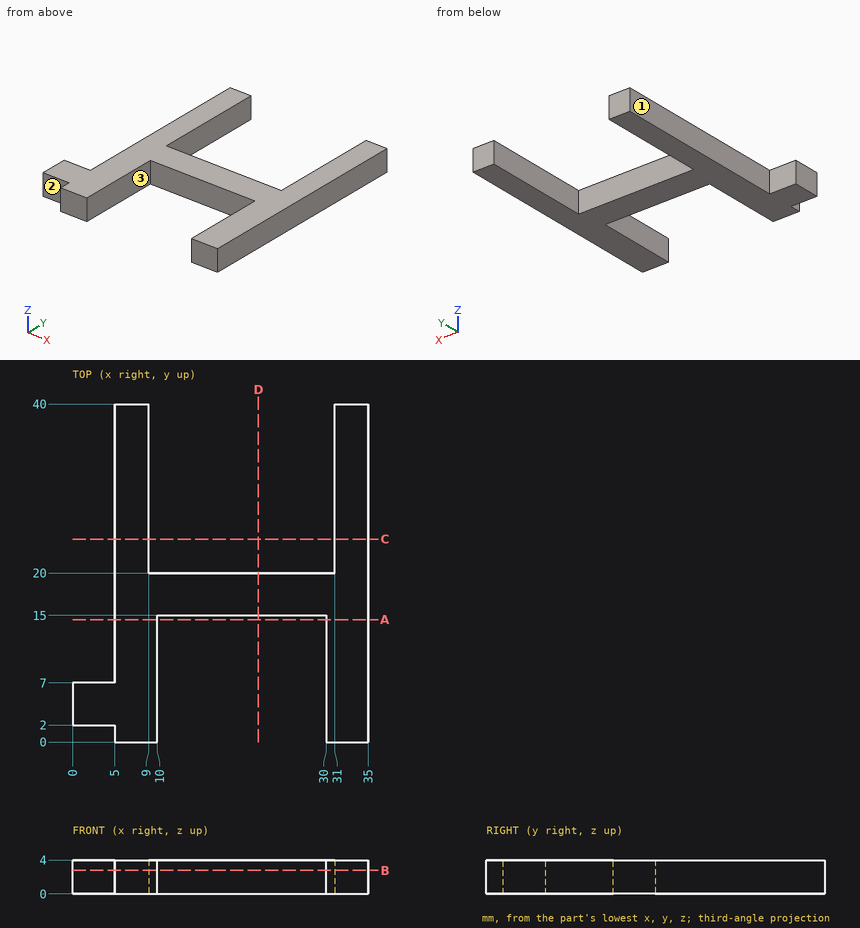
Drawing for the job (mm, zero at the part's lowest x, y, z). A direction names the side the tool comes from. Round coordinates to 2 decimals unless told otherwise and drop trailing zeros. Loops run counter-clockwise (first coordinate to the right, second up) from the corner with the lowest first, then second, coordinate; pieces in that order, holes last. Notation, with made-up numbers: (31.5, 30.25) - (82.5, 30.25) arc R24 ccw to (82.5, 47.25) - close; hole circle Ø10 at (-30, -27). An arc over 180 degrees is marked (long way). Return JSON: item names as keys, results as strings. Group by question number.
Q1. Band-saw the part on A-A on y = 14.5. Give the cut face in (x, z), plus the area to 3 significant figures.
Q2. Band-saw the part on B-B on z = 2.8. Give the cut face in (x, y), plus the area to 3 significant figures.
Q3. Flat gauge pins, fed straight in: pin 1 Ø1 at (y, z) = (1, 3) entering from -X; pin 2 Ø12 at (x, y) = (30, 13.5) entering from -Z; pin 3 Ø2 at (x, z) = (16, 1.5) entering from -Y; pin 4 Ø1.5 at (x, y) = (10, 21.5) entering from -Z. Where does each tip first touch, or does it go through?
Q4. Band-saw the part on C-C on y = 24. Give the cut face in (x, z), plus the area to 3 significant figures.
Q5. Tool access for the marked faces 1, 2 and 3: list every direction of +Z, -Z, +X, -X, +Y, -Y with a clear straight run to the whole face (end or side of a thin tool).
Q6. Drill centre lines: line 1 along X through (y, z) = (29.5, 2.75); line 2 along X through (y, z) = (2.5, 2.9); line 3 along X through (y, z) = (19, 2.7). Where is each one in solid material? Low to high. Write a range as [from, to].
Q7. Band-saw the part on D-D on x = 22. Give the cut face in (y, z), plus the area to 3 significant figures.
Solutions:
{
 "1": {"outline": "(5, 0) - (10, 0) - (10, 4) - (5, 4) - close; (30, 0) - (35, 0) - (35, 4) - (30, 4) - close", "area": "40.0 mm^2"},
 "2": {"outline": "(0, 2) - (5, 2) - (5, 0) - (10, 0) - (10, 15) - (30, 15) - (30, 0) - (35, 0) - (35, 40) - (31, 40) - (31, 20) - (9, 20) - (9, 40) - (5, 40) - (5, 7) - (0, 7) - close", "area": "485 mm^2"},
 "3": {"pin 1": "stops at x = 5", "pin 2": "stops at z = 0", "pin 3": "stops at y = 15", "pin 4": "passes through"},
 "4": {"outline": "(5, 0) - (9, 0) - (9, 4) - (5, 4) - close; (31, 0) - (35, 0) - (35, 4) - (31, 4) - close", "area": "32.0 mm^2"},
 "5": {"face 1": "+Z, -Z, -X, +Y", "face 2": "+Z, -Z, -X, -Y", "face 3": "+Z, -Z, -Y"},
 "6": {"line 1": "x = [5, 9], [31, 35]", "line 2": "x = [0, 10], [30, 35]", "line 3": "x = [5, 35]"},
 "7": {"outline": "(15, 0) - (20, 0) - (20, 4) - (15, 4) - close", "area": "20.0 mm^2"}
}
